from build123d import *

# Parameters (mm, degrees)
ESQUISSE2_R             = 6
ENL_V_MAT_EXTRU_1_DEPTH = 40


with BuildPart() as part:
    # Esquisse1 → Révolution1 (revolve)
    with BuildSketch(Plane.XY, mode=Mode.PRIVATE) as r_volution1_sk:
        Polygon((-55.657677475, 42), (-53.657677475, 42), (-45.730447287, 25), (-25.584907664, 25), (-17.657677475, 42), (-15.657677475, 42), (-15.657677475, 18), (-5.657677475, 18), (-5.657677475, 3), (-65.657677475, 3), (-65.657677475, 18), (-55.657677475, 18), align=None)
    revolve(r_volution1_sk.sketch.rotate(Axis((-128.723358614, 0, 0), (1, 0, 0)), 90), axis=Axis((-128.723358614, 0, 0), (1, 0, 0)))  # turned: the seam where the file's is

    # Esquisse2 → Enlèv. mat.-Extru.1 (cut)
    with BuildSketch(Plane(origin=(-5.657677475, 0, 0), x_dir=(0, 0, -1), z_dir=(1, 0, 0))):
        Circle(ESQUISSE2_R)
    extrude(amount=-ENL_V_MAT_EXTRU_1_DEPTH, mode=Mode.SUBTRACT)


solid = part.part
For this review, take the finished solid that the model builds, in its own axes (mm). A direction names the side the tool comes from. Round coordinates to 2 decimals unless told otherwise and drop trailing zeros. Order: outer loops, then holes, each group sorted by start corner. A loop starts at its lowest first (then second) coordinate and runs counter-clockwise, first axis right, second up. Notation, with made-up numbers: (22, 17) -> (75, 17) arc R31 ccw to (75, 56) -> close; hole circle Ø10 at (-15.75, 56). An arc over 180 degrees is marked (long way). Write item = value, one per line. Start each with the question number.
1) Take a section at A-A on z = 0. State the section outline as (x, y) points.
2) To check wall thickness, follow line 1 (Y direction, x = -31.5, z = 0); line 2 (Y direction, x = -55.25, z = 0); line 3 (X direction, y = -1.5, z = 20). State the ranges of each line that lie inside material, in increasing order. Write a range as from..to.
3) Take a section at B-B on x = -37. State the section outline as (y, z) points.
4) The part is to be moulded in two halves that separate along X. For faces 6 (the face through (-46.115, 15.714, -20.494)), 7 (the face through (-60.588, -12.165, -13.267)), 8 (the face through (-25.09, -7.83, 24.86)), 9 (the face through (-45.658, -1, 3)), say which applies: +X half, -X half, draft (parallel to the pull), parting line (faces both ways), or undercut.
5) Insertion check: pin 1 (12 mm diameter, centred on x = -35, y = 6, fed in from -Z); pin 2 (8 mm diameter, centred on x = -28.5, z = -2.5, fed in from -Y); pin 3 (4 mm diameter, centred on x = -55, z = -6, fed in from +Y). Each pin has a flat end and moves straight along its axis. Give the tip position at first contact, or say it passes through.
6) Tool access review of faces 1 (the face through (-55.658, 9, -18)), 2 (the face through (-35.517, -7.509, 23.846)), 3 (the face through (-10.588, -12.165, -13.267)), 4 (the face through (-5.658, 8, 0)), 5 (the face through (-55.8, -0.9, 2.86)): name each direction out of +Z, -Z, +X, -X, +Y, -Y from which nothing blocks a thin tool from reaching the whole face with its end or side.
7) Take a section at C-C on x = -19.5. State the section outline as (y, z) points.
Verdict:
q1.outline = (-65.66, -18) -> (-55.66, -18) -> (-55.66, -42) -> (-53.66, -42) -> (-45.73, -25) -> (-25.58, -25) -> (-17.66, -42) -> (-15.66, -42) -> (-15.66, -18) -> (-5.66, -18) -> (-5.66, -6) -> (-45.66, -6) -> (-45.66, -3) -> (-65.66, -3) -> close; (-65.66, 3) -> (-45.66, 3) -> (-45.66, 6) -> (-5.66, 6) -> (-5.66, 18) -> (-15.66, 18) -> (-15.66, 42) -> (-17.66, 42) -> (-25.58, 25) -> (-45.73, 25) -> (-53.66, 42) -> (-55.66, 42) -> (-55.66, 18) -> (-65.66, 18) -> close
q2.line_1 = -25..-6, 6..25
q2.line_2 = -42..-3, 3..42
q2.line_3 = -55.66..-15.66
q3.outline = circle Ø50 at (0, 0); hole circle Ø12 at (0, 0)
q4.face_6 = undercut
q4.face_7 = draft
q4.face_8 = undercut
q4.face_9 = +X half
q5.pin_1 = -25
q5.pin_2 = -27.22
q5.pin_3 = 41.81
q6.face_1 = -X
q6.face_2 = none
q6.face_3 = +X
q6.face_4 = +Z, -Z, +X, +Y, -Y
q6.face_5 = +X, -X
q7.outline = circle Ø76.1 at (0, 0); hole circle Ø12 at (0, 0)
